from build123d import *

# Parameters (mm, degrees)
EXTRUDE_1_DEPTH     = 11.5
FILLET_1_R          = 2
FILLET_2_R          = 1.5
SKETCH_2_R          = 1
CUT_EXTRUDE_1_DEPTH = 11.5


with BuildPart() as part:
    # 草图1 → 凸台-拉伸1 (new body)
    with BuildSketch(Plane.XY):
        Polygon((0, 0), (0, 9.85), (11.8, 9.85), (11.8, 0), (17.3, 0), (17.3, 3.2), (13.1, 3.2), (13.1, 11.5), (-1.3, 11.5), (-1.3, 3.2), (-5.5, 3.2), (-5.5, 0), align=None)
    extrude(amount=EXTRUDE_1_DEPTH)

    # 圆角1
    fillet_1_edges = [part.edges().sort_by_distance(p)[0] for p in [
        (11.8, 9.85, 5.75),
        (0, 9.85, 5.75),
    ]]
    fillet(fillet_1_edges, radius=FILLET_1_R)

    # 圆角2
    fillet_2_edges = [part.edges().sort_by_distance(p)[0] for p in [
        (-1.3, 11.5, 5.75),
        (13.1, 11.5, 5.75),
    ]]
    fillet(fillet_2_edges, radius=FILLET_2_R)

    # 草图2 → 切除-拉伸1 (cut)
    with BuildSketch(Plane(origin=(0, 3.2, 0), x_dir=(1, 0, 0), z_dir=(0, 1, 0))):
        with Locations((-2.9, -4.2)):
            Circle(SKETCH_2_R)
        with Locations((14.7, -4.2)):
            Circle(SKETCH_2_R)
    extrude(amount=-CUT_EXTRUDE_1_DEPTH, mode=Mode.SUBTRACT)


solid = part.part
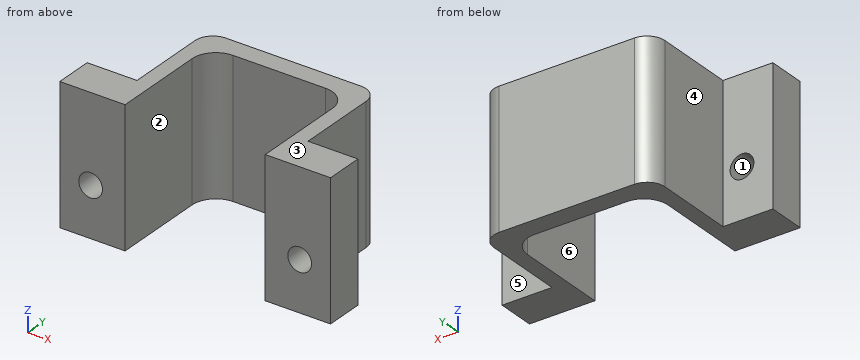
Geometry: final body of the model. Coordinates: model frame, mm. Face numbers are marked on the shaded views. A direction names the side the tool comes from. Round coordinates to 2 decimals unless told otherwise and drop trailing zeros. Order: outer loops, then holes, each group sorted by start corner. A loop starts at its lowest first (then second) coordinate and runs counter-clockwise, first axis right, second up. Notation, with made-up numbers: (-36.5, 9.5) - (-14.5, 9.5) arc R29 cw to (-14.5, 35.5) - close; hole circle Ø11 at (-1, -15.75). An arc over 180 degrees is marked (long way). Write each question's results on one line, items separated by ' | '.
Item 1: Section C-C, the plane y = 7.5. Return the cut outline in (x, z).
Completed:
outline: (-1.3, 0) - (0, 0) - (0, 11.5) - (-1.3, 11.5) - close; (11.8, 0) - (13.1, 0) - (13.1, 11.5) - (11.8, 11.5) - close
Item 2: Reachability of the marked faces 4, 5 and 6 from +Z, -Z, +X, -X, +Y, -Y: full face, straight path, thin tool, end or side. Return the list, or none.
Completed:
face 4: +Z, -Z, -X, +Y | face 5: +Z, -Z, +X, +Y | face 6: +Z, -Z, -Y
Item 3: Mould query, pull axis Z, two halves, no side actions, for the marked faces 1, 2 and 3. Classes: pulls with the +Z half, pulls with the -Z half, needs draft (parallel to the pull), parting line crosses it, or undercut.
Completed:
face 1: undercut | face 2: needs draft | face 3: pulls with the +Z half
Item 4: Section B-B, the plane z = 4.2. Return the cut outline in (x, y).
Completed:
outline: (-5.5, 0) - (-3.9, 0) - (-3.9, 3.2) - (-5.5, 3.2) - close; (-1.9, 0) - (0, 0) - (0, 7.85) arc R2 cw to (2, 9.85) - (9.8, 9.85) arc R2 cw to (11.8, 7.85) - (11.8, 0) - (13.7, 0) - (13.7, 3.2) - (13.1, 3.2) - (13.1, 10) arc R1.5 ccw to (11.6, 11.5) - (0.2, 11.5) arc R1.5 ccw to (-1.3, 10) - (-1.3, 3.2) - (-1.9, 3.2) - close; (15.7, 0) - (17.3, 0) - (17.3, 3.2) - (15.7, 3.2) - close
Item 5: Section A-A, the plane x = -2.9. Return the cut outline in (y, z).
Completed:
outline: (0, 0) - (3.2, 0) - (3.2, 3.2) - (0, 3.2) - close; (0, 5.2) - (3.2, 5.2) - (3.2, 11.5) - (0, 11.5) - close
Item 6: First-contact query: pin 1 Ø2 at (y, z) = (8, 8.5) entering from -X; pin 2 Ø3 at (x, z) = (-2.9, 4.2) entering from +Y; pin 3 Ø2 at (y, z) = (8, 7.5) entering from +X; pin 4 Ø1.2 at (x, z) = (14.7, 4.2) entering from -Y. Flat tips, straight axial feed; report the tip coordinate or a pass-through.
Completed:
pin 1: x = -1.3 | pin 2: y = 3.2 | pin 3: x = 13.1 | pin 4: through
Item 7: Material intervals for line 1 along X through (y, z) = (2.4, 4.2); line 2 along Z through (x, y) = (14.7, 1.1); line 3 along X through (y, z) = (1.5, 7), sorted ascending. Write a range as [from, to].
Completed:
line 1: [-5.5, -3.9], [-1.9, 0], [11.8, 13.7], [15.7, 17.3] | line 2: [0, 3.2], [5.2, 11.5] | line 3: [-5.5, 0], [11.8, 17.3]
Item 8: Section D-D, the plane z = 2.25. Return the cut outline in (x, y), and give its area (3 significant figures).
Completed:
outline: (-5.5, 0) - (0, 0) - (0, 7.85) arc R2 cw to (2, 9.85) - (9.8, 9.85) arc R2 cw to (11.8, 7.85) - (11.8, 0) - (17.3, 0) - (17.3, 3.2) - (13.1, 3.2) - (13.1, 10) arc R1.5 ccw to (11.6, 11.5) - (0.2, 11.5) arc R1.5 ccw to (-1.3, 10) - (-1.3, 3.2) - (-5.5, 3.2) - close | area: 77.0 mm^2
